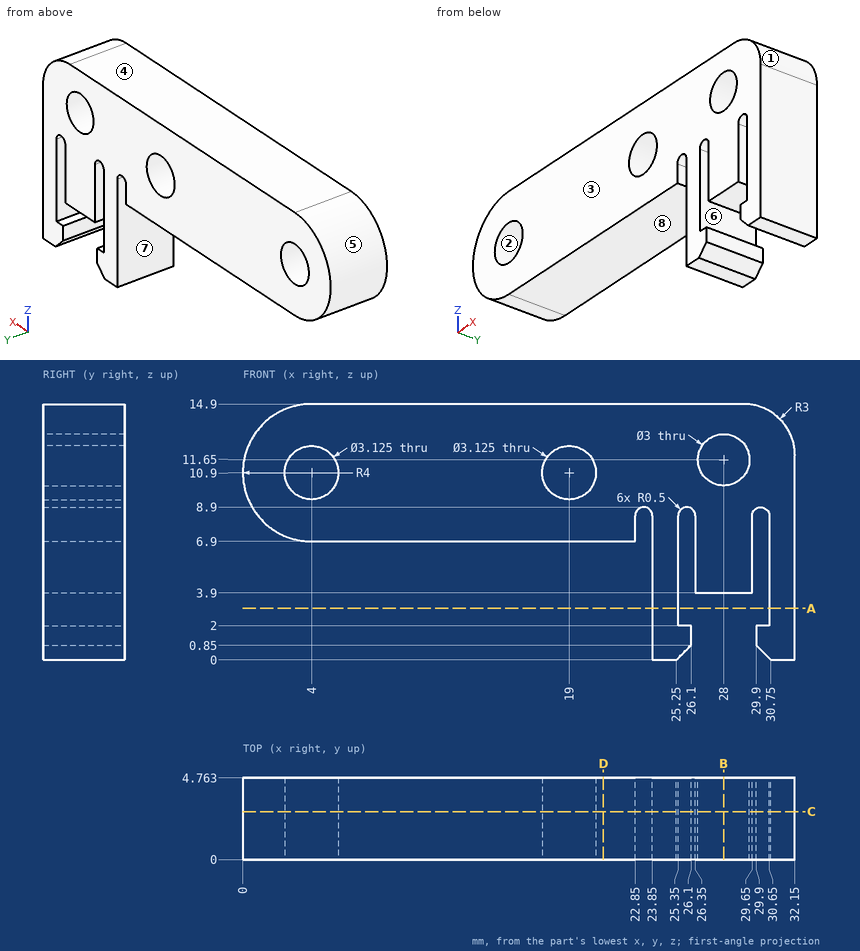
Study the drawing (mm; zero at the part's minimum x, y, z) and answer. A direction names the side the tool comes from. Give positions to 0.01 mm unless a question says otherwise; leave off trailing zeros. Write each loop counter-clockwise with the first axis right and the second up, starting at its lowest first coordinate (ties: lowest second). Pieces come first, ordered by that corner, then holes. Notation, with made-up numbers: M 72.25,45 L 127.25,45 A17 cw 127.25,53 Z; hole C 45.25,55 d7. An arc over 180 degrees is marked long. Put each result on its own line as item: value. Start each with the question number.
1. Which of the six approach directions +Z, -Z, +X, -X, +Y, -Y give full straight-line access (tool end or side, diameter ignored) to the marked faces 4, 5, 6, 7 and 8?
2. For a pull along X with two mould halves and no side action, classify the marked faces 1, 2 and 3 as released by +X, released by -X, zero draft, split by the parting line, or undercut.
3. The part is cut by section A-A, the plane z = 3. Give the vertices of the cut face in (x, y), and give its area (3 significant figures).
4. The part is cut by section B-B, the plane x = 28. Give the vertices of the cut face in (y, z), and give its area (3 significant figures).
5. Consider line 1 along X through (y, z) = (2.8, 4.75); line 2 along X through (y, z) = (2.35, 2.5); line 3 along X through (y, z) = (1.75, 1.5). Determine where each line is inside the solid, lowest interval first.
6. The part is cut by section C-C, the plane y = 2.8. Give the number of separate pieces and of enclosed holes in the cut face, and give its area (3 significant figures).
7. Each of these flat-tipped pins is pushed along its axis until it touches: pin 1 Ø1.5 at (x, z) = (15, 8.5) entering from -Y; pin 2 Ø1.4 at (y, z) = (3, 4) entering from -X; pin 3 Ø1.4 at (y, z) = (2.5, 6.5) entering from -X; pin 4 Ø2.5 at (x, y) = (10.5, 2.5) entering from -Z. Where does it stop, or does it pass through?
8. The part is cut by section D-D, the plane x = 21. Give the vertices of the cut face in (y, z), and give its area (3 significant figures).
Final values:
1. face 4: +Z, +X, -X, +Y, -Y
1. face 5: -X, +Y, -Y
1. face 6: +Y, -Y
1. face 7: -Z, +Y, -Y
1. face 8: -Z, -X, +Y, -Y
2. face 1: released by +X
2. face 2: undercut
2. face 3: zero draft
3. outline: M 23.85,0 L 25.35,0 L 25.35,4.76 L 23.85,4.76 Z; M 30.65,0 L 32.15,0 L 32.15,4.76 L 30.65,4.76 Z
3. area: 14.3 mm²
4. outline: M 0,3.9 L 4.76,3.9 L 4.76,10.15 L 0,10.15 Z; M 0,13.15 L 4.76,13.15 L 4.76,14.9 L 0,14.9 Z
4. area: 38.1 mm²
5. line 1: x = 23.85 to 25.35, 26.35 to 29.65, 30.65 to 32.15
5. line 2: x = 23.85 to 25.35, 30.65 to 32.15
5. line 3: x = 23.85 to 26.1, 29.9 to 32.15
6. separate pieces: 1
6. enclosed holes: 3
6. area: 253 mm²
7. pin 1: stops at y = 0
7. pin 2: stops at x = 23.85
7. pin 3: stops at x = 2.48
7. pin 4: stops at z = 6.9
8. outline: M 0,6.9 L 4.76,6.9 L 4.76,14.9 L 0,14.9 Z
8. area: 38.1 mm²
